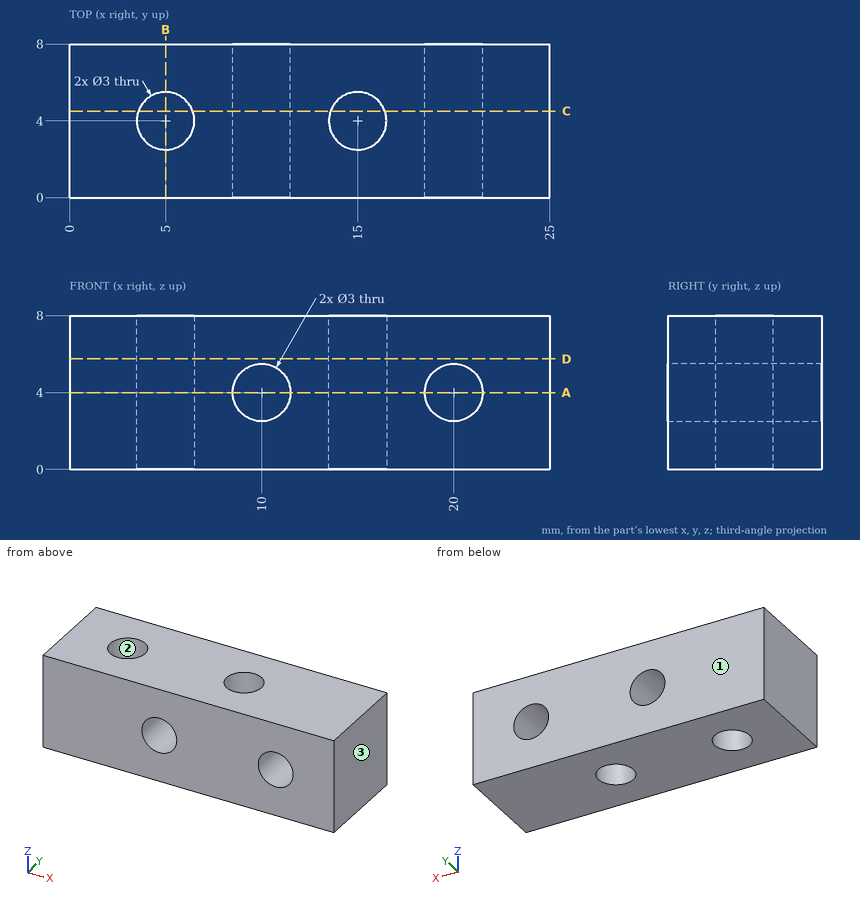
Input: dimensioned drawing with shaded views. Units: mm. Origin: part minimum x, y, z. Give positions to 0.01 mm unless a question says otherwise; leave off trailing zeros. Write each loop counter-clockwise with the first axis right and the second up, starting at its lowest first coordinate (ties: lowest second). Pieces come first, ordered by that corner, then holes.
1. Material intervals for line 1 along X through (y, z) = (3.75, 6.5); line 2 along X through (y, z) = (0.5, 5); line 3 along X through (y, z) = (4.5, 4), sorted ascending.
2. Section query A-A (z = 4). Return the cut outline in (x, y), then the cut area to 3 significant figures.
3. Section query D-D (z = 5.75). Return the cut outline in (x, y), then the cut area to 3 significant figures.
4. Section query C-C (y = 4.5). Return the cut outline in (x, z).
5. Section query B-B (x = 5). Return the cut outline in (y, z), then the cut area to 3 significant figures.
6. Pull-direction query (Y, two-part tool) for the marked faces 1, 2 and 3; classes: +Y half, -Y half, draft (parallel to the pull), parting line (faces both ways), or undercut.
Output values:
1. line 1: x = 0 to 3.52, 6.48 to 13.52, 16.48 to 25
1. line 2: x = 0 to 8.88, 11.12 to 18.88, 21.12 to 25
1. line 3: x = 0 to 3.59, 6.41 to 8.5, 11.5 to 13.59, 16.41 to 18.5, 21.5 to 25
2. outline: (0, 0) - (8.5, 0) - (8.5, 8) - (0, 8) - close; (11.5, 0) - (18.5, 0) - (18.5, 8) - (11.5, 8) - close; (21.5, 0) - (25, 0) - (25, 8) - (21.5, 8) - close; hole circle Ø3 at (5, 4); hole circle Ø3 at (15, 4)
2. area: 138 mm2
3. outline: (0, 0) - (25, 0) - (25, 8) - (0, 8) - close; hole circle Ø3 at (5, 4); hole circle Ø3 at (15, 4)
3. area: 186 mm2
4. outline: (0, 0) - (3.59, 0) - (3.59, 8) - (0, 8) - close; (6.41, 0) - (13.59, 0) - (13.59, 8) - (6.41, 8) - close; (16.41, 0) - (25, 0) - (25, 8) - (16.41, 8) - close; hole circle Ø3 at (10, 4); hole circle Ø3 at (20, 4)
5. outline: (0, 0) - (2.5, 0) - (2.5, 8) - (0, 8) - close; (5.5, 0) - (8, 0) - (8, 8) - (5.5, 8) - close
5. area: 40.0 mm2
6. face 1: +Y half
6. face 2: undercut
6. face 3: draft
